Autodesk Fusion 360 part; units mm, degrees
sketch "Sketch1" plane through (0, 0, 0) normal (0, 1, 0) x (1, 0, 0)
  line L0 (2, 0) -> (20, 0)
  line L1 (20, 0) -> (20, -10)
  line L2 (20, -10) -> (2, -10)
  line L3 (0, -8) -> (0, -2)
  arc A0 (2, 0) -> (0, -2) centre (2, -2) ccw
  arc A1 (0, -8) -> (2, -10) centre (2, -8) ccw
  point P0 (0, -10)
  dimension "d1" = 10
  dimension "d2" = 20
  dimension "d12" = 2
extrude "Extrude1" add sketch "Sketch1" along normal blind 3
sketch "Sketch2" plane through (0, 3, 0) normal (0, 1, 0) x (-1, 0, 0)
  line L0 (-2, 10) -> (-20, 10)
  line L1 (-20, 10) -> (-20, 0)
  line L2 (-20, 0) -> (-2, 0)
  line L3 (0, 2) -> (0, 8)
  line L4 (-3, 9) -> (-19, 9)
  line L5 (-19, 9) -> (-19, 1)
  line L6 (-19, 1) -> (-3, 1)
  line L7 (-1, 3) -> (-1, 7)
  circle A0 centre (-4, 5) radius 1.5
  line L8 (0, 5) -> (-20, 5) construction
  line L9 (-11, 0) -> (-11, 10) construction
  arc A1 (-2, 0) -> (0, 2) centre (-2, 2) ccw
  arc A2 (0, 8) -> (-2, 10) centre (-2, 8) ccw
  arc A3 (-3, 1) -> (-1, 3) centre (-3, 3) ccw
  arc A4 (-1, 7) -> (-3, 9) centre (-3, 7) ccw
  dimension "d6" = 3
  dimension "d7" = 3
  dimension "d13" = 2
  dimension "d14" = 2
extrude "Extrude2" add sketch "Sketch2" along normal blind 1 contours L0 L1 L2 L3 A1 A2
extrude "Extrude3" cut sketch "Sketch2" against normal blind 3 contours A0
Check sheet for the modelled part. Datum: model origin and axes. Units: mm. A direction names the side the tool comes from. Give positions to 0.01 mm unless a question says otherwise; leave off trailing zeros. Order: outer loops, then holes, each group sorted by start corner. A loop starts at its lowest first (then second) coordinate and runs counter-clockwise, first axis right, second up. Notation, with made-up numbers: M 62,46.5 L 97,46.5 A21 cw 97,80.5 Z; hole C 78.25,-7 d4. An arc over 180 degrees is marked long. Answer as CSV lines item,"result". Start each with the question number.
Item 1: Cross-section at C-C on y = 0.3. Enter the section's corners in (x, z), plus the area to 3 significant figures.
Item 2: Mould release check, pull along Z, two halves, no side actions. Record for faces 1 (the face through (0.57, 1.97, 0.6)), 2 (the face through (0.6, 1.97, 9.43)), 3 (the face through (2.614, 1.521, 4.425)): +Z half, -Z half, draft (parallel to the pull), parting line (faces both ways), or undercut.
Item 3: Thickness scan on line 1 (X direction, y = 3.5, z = 5.5); line 2 (Z direction, x = 4, y = 1.9); line 3 (Z direction, x = 6, y = 3.3). Record the ranges inside material, lowest first. Write a range as [from, to].
Item 4: Gauge pin test, flat ends, axial feed: P1, Ø2.5, axis at x = 4, z = 5, coming from the -Y side; P2, Ø2.5, axis at x = 11, z = 5.5, coming from the +Y side. Record the tip position at first contact, or that the pin passes through.
Item 5: Tool access check on faces 4 (the face through (11, 2, 0)), 5 (the face through (10, 3, 5)). Record the directions out of +Z, -Z, +X, -X, +Y, -Y that give a thin tool (end or side, any length) a straight path to the whole face; none if there is none.
Item 6: Cross-section at A-A on x = 4. Enter the section's corners in (y, z).
Item 7: Cross-section at B-B on z = 5. Enter the section's corners in (x, y), plus the area to 3 significant figures.
Item 8: Cross-section at D-D on x = 17.5. Enter the section's corners in (y, z).
Established:
1,outline,"M 0,2 A2 ccw 2,0 L 20,0 L 20,10 L 2,10 A2 ccw 0,8 Z; hole C 4,5 d3"
1,area,"191 mm^2"
2,face 1,"-Z half"
2,face 2,"+Z half"
2,face 3,"undercut"
3,line 1,"x = [0, 1], [19, 20]"
3,line 2,"z = [0, 3.5], [6.5, 10]"
3,line 3,"z = [0, 1], [9, 10]"
4,P1,"passes through"
4,P2,"stops at y = 3"
5,face 4,"-Z, +X, -X, +Y, -Y"
5,face 5,"+Y"
6,outline,"M 0,0 L 4,0 L 4,1 L 3,1 L 3,3.5 L 0,3.5 Z; M 0,6.5 L 3,6.5 L 3,9 L 4,9 L 4,10 L 0,10 Z"
7,outline,"M 0,0 L 2.5,0 L 2.5,3 L 1,3 L 1,4 L 0,4 Z; M 5.5,0 L 20,0 L 20,4 L 19,4 L 19,3 L 5.5,3 Z"
7,area,"53.0 mm^2"
8,outline,"M 0,0 L 4,0 L 4,1 L 3,1 L 3,9 L 4,9 L 4,10 L 0,10 Z"
